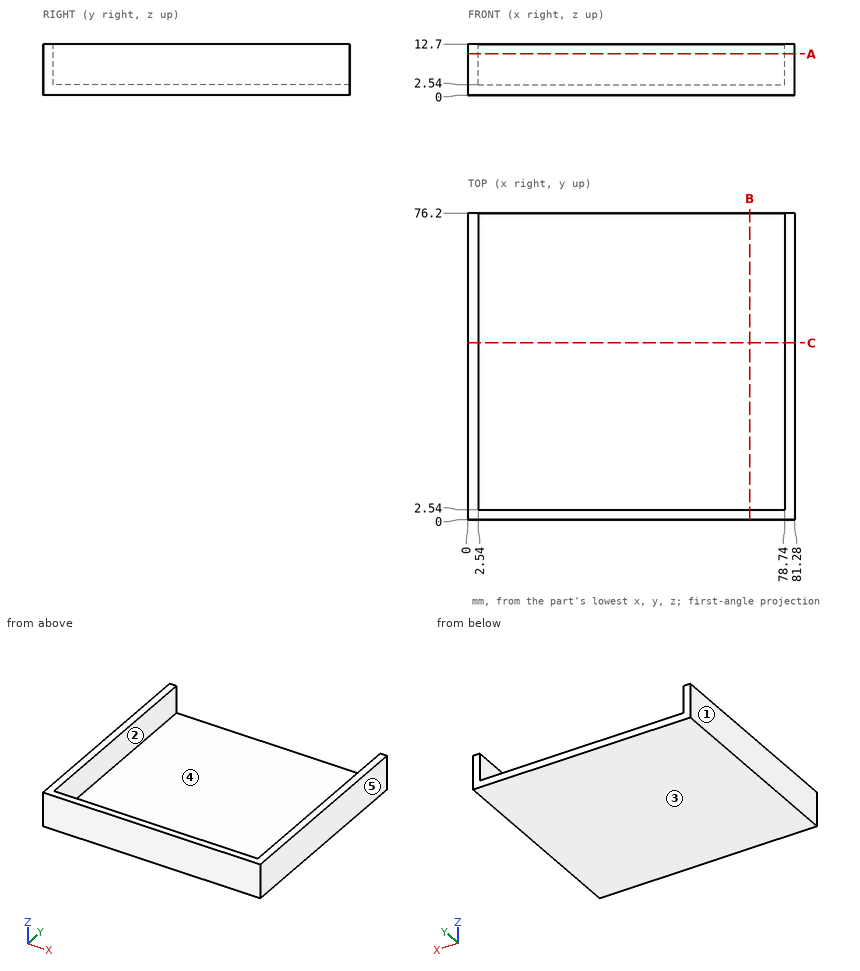
Input: dimensioned drawing with shaded views. Units: mm. Origin: part minimum x, y, z. A direction names the side the tool comes from. Give positions to 0.01 mm unless a question says otherwise; leave off trailing zeros. Loops run counter-clockwise (first coordinate to the right, second up) from the corner with the lowest first, then second, coordinate; pieces in that order, holes last. Notation, with made-up numbers: (-36.5, 55.5) -> (21.5, 55.5) arc R31 ccw to (21.5, 92.5) -> close; hole circle Ø11 at (18.25, -12.75). An arc over 180 degrees is marked (long way). Use a Markdown table: item, result.
Q1. First-contact query: P1, Ø6, axis at x = 39.5, z = 10, coming from the +Y side; P2, Ø10, axis at x = 9.5, y = 49, coming from the +Z side. Flat tips, straight axial feed; report the tip coordinate or a pass-through.
Entries:
| item | result |
|---|---|
| P1 | stops at y = 2.54 |
| P2 | stops at z = 2.54 |
Q2. Access query for the marked faces 4 and 5. Directions: +Z, -Z, +X, -X, +Y, -Y. A direction counts if a zero-diameter tool reaches every point of the face in a straight line with its end or side. Return the directions, or none.
Entries:
| item | result |
|---|---|
| face 4 | +Z, +Y |
| face 5 | +Z, -Z, +X, +Y, -Y |
Q3. Section query C-C, the plane y = 44. Return the cut outline in (x, z).
Entries:
| item | result |
|---|---|
| outline | (0, 0) -> (81.28, 0) -> (81.28, 12.7) -> (78.74, 12.7) -> (78.74, 2.54) -> (2.54, 2.54) -> (2.54, 12.7) -> (0, 12.7) -> close |
Q4. Section query A-A, the plane z = 10.25. Return the cut outline in (x, y), plus the area to 3 significant figures.
Entries:
| item | result |
|---|---|
| outline | (0, 0) -> (81.28, 0) -> (81.28, 76.2) -> (78.74, 76.2) -> (78.74, 2.54) -> (2.54, 2.54) -> (2.54, 76.2) -> (0, 76.2) -> close |
| area | 581 mm² |
Q5. Section query B-B, the plane x = 70. Return the cut outline in (y, z), plus the area to 3 significant figures.
Entries:
| item | result |
|---|---|
| outline | (0, 0) -> (76.2, 0) -> (76.2, 2.54) -> (2.54, 2.54) -> (2.54, 12.7) -> (0, 12.7) -> close |
| area | 219 mm² |
Q6. Ray query, probe 1 along X at (y, z) = (50, 8.5); probe 2 along Z at (x, y) = (8, 50). Return the intervals inside material, ascending. Write a range as from..to.
Entries:
| item | result |
|---|---|
| probe 1 | x = 0..2.54, 78.74..81.28 |
| probe 2 | z = 0..2.54 |
Q7. Pull-direction query (X, two-part tool) for the marked faces 1, 2 and 3; classes: pulls with the +X half, pulls with the -X half, needs draft (parallel to the pull), parting line crosses it, or undercut.
Entries:
| item | result |
|---|---|
| face 1 | pulls with the -X half |
| face 2 | undercut |
| face 3 | needs draft |
